from build123d import *

# Parameters (mm, degrees)
EXTRUDE_1_DEPTH          = 170
SKETCH_2_R               = 60
CUT_EXTRUDE_1_DEPTH      = 180
CUT_EXTRUDE_2_DEPTH      = 313.955268369
CUT_EXTRUDE_2_DEPTH_BACK = 313.955268369
SKETCH_3_R               = 30
FILLET_1_R               = 70
FILLET_2_R               = 20
FILLET_3_R               = 20


with BuildPart() as part:
    # 草图1 → 凸台-拉伸1 (new body)
    with BuildSketch(Plane.XY):
        Polygon((-180, 0), (0, 0), (0, -175), (8, -175), (8, 8), (-180, 8), (-188, 8), (-188, -175), (-180, -175), align=None)
    extrude(amount=EXTRUDE_1_DEPTH)

    # 草图2 → 切除-拉伸1 (cut)
    with BuildSketch(Plane(origin=(0, 8, 0), x_dir=(1, 0, 0), z_dir=(0, 1, 0))):
        with Locations(Location((-90, -85, 0), (0, 0, 180))):
            Circle(SKETCH_2_R)
    extrude(amount=-CUT_EXTRUDE_1_DEPTH, mode=Mode.SUBTRACT)

    # 草图3 → 切除-拉伸2 (cut, two sides: drawn at the far end of the back side and taken through both)
    with BuildSketch(Plane(origin=(8, 0, 0), x_dir=(0, 0, -1), z_dir=(1, 0, 0)).offset(-CUT_EXTRUDE_2_DEPTH_BACK)):
        with Locations(Location((-85, -95, 0), (0, 0, 90))):
            Circle(SKETCH_3_R)
    extrude(amount=CUT_EXTRUDE_2_DEPTH + CUT_EXTRUDE_2_DEPTH_BACK, mode=Mode.SUBTRACT)

    # 圆角1
    fillet_1_edges = [part.edges().sort_by_distance(p)[0] for p in [
        (4, -175, 0),
        (4, -175, 170),
        (-184, -175, 170),
        (-184, -175, 0),
    ]]
    fillet(fillet_1_edges, radius=FILLET_1_R)

    # 圆角2
    fillet_2_edges = [part.edges().sort_by_distance(p)[0] for p in [
        (0, 0, 85),
        (-180, 0, 85),
    ]]
    fillet(fillet_2_edges, radius=FILLET_2_R)

    # 圆角3
    fillet_3_edges = [part.edges().sort_by_distance(p)[0] for p in [
        (-188, 8, 85),
        (8, 8, 85),
    ]]
    fillet(fillet_3_edges, radius=FILLET_3_R)


solid = part.part
Build history of the part. All positions in model axes, mm. A direction names the side the tool comes from. Coordinates: 2 decimals unless noted, no trailing zeros. Order: outer loops, then holes, each group sorted by start corner. A loop starts at its lowest first (then second) coordinate and runs counter-clockwise, first axis right, second up. Notation, with made-up numbers: (61, -35) - (75, -35) arc R24 ccw to (75, -13) - close; hole circle Ø4 at (2, -3). An arc over 180 degrees is marked (long way). Write item = value, one per line. Start each with the question number.
1) Saw through at B-B on y = -95. Write the cut outline in (x, z), then the cut area to 3 significant figures.
2) Flat gauge pin, fed straight in: pin 1 Ø3 at (x, z) = (-150, 111.5) entering from -Y. Where does the tip first touch, or does it go through?
3) Saw through at C-C on y = -24. Write the cut outline in (x, z), then the cut area to 3 significant figures.
4) 3-axis set-ups, long thin cutter, end or side, ignore diameter. For faces 4 (the face through (-183.94, -153.95, 19.96)), 5 (the face through (-6.014, -5.703, 86.19)): which of +Z, -Z, +X, -X, +Y, -Y reach the whole face in a straight line?
5) Saw through at D-D on x = -90. Write the cut outline in (y, z), then the cut area to 3 significant figures.
6) Wall check: line 1 along Z through (x, y) = (-186, -95); line 2 along X through (y, z) = (-96, 120); line 3 along X through (y, z) = (-15.5, 33). Give the ranges that are in metal, low to high. Write a range as from..to.
7) Saw through at A-A on z = 85. Write the cut outline in (x, y).
8) Two-plate mould, pull along Y, no slides. Class faces 1 (the face through (-107, 0, 27)), 2 (the face through (-184.056, -117.111, 105.275)), 3 (the face through (0, -62, 84)): pulls with the +Y half, pulls with the -Y half, needs draft (parallel to the pull), parting line crosses it, or undercut.
From the geometry:
q1.outline = (-188, 0) - (-180, 0) - (-180, 55) - (-188, 55) - close; (-188, 115) - (-180, 115) - (-180, 170) - (-188, 170) - close; (0, 0) - (8, 0) - (8, 55) - (0, 55) - close; (0, 115) - (8, 115) - (8, 170) - (0, 170) - close
q1.area = 1,760 mm^2
q2.pin_1 = 0
q3.outline = (-188, 0) - (-180, 0) - (-180, 170) - (-188, 170) - close; (0, 0) - (8, 0) - (8, 170) - (0, 170) - close
q3.area = 2,720 mm^2
q4.face_4 = -Z, +X, -X, -Y
q4.face_5 = +Z, -Z, -Y
q5.outline = (0, 0) - (8, 0) - (8, 25) - (0, 25) - close; (0, 145) - (8, 145) - (8, 170) - (0, 170) - close
q5.area = 400 mm^2
q6.line_1 = 0..55, 115..170
q6.line_2 = -188..-180, 0..8
q6.line_3 = -188..-179.49, -0.51..8
q7.outline = (-188, -175) - (-180, -175) - (-180, -125) - (-188, -125) - close; (-188, -65) - (-180, -65) - (-180, -20) arc R20 cw to (-160, 0) - (-150, 0) - (-150, 8) - (-168, 8) arc R20 ccw to (-188, -12) - close; (-30, 0) - (-20, 0) arc R20 cw to (0, -20) - (0, -65) - (8, -65) - (8, -12) arc R20 ccw to (-12, 8) - (-30, 8) - close; (0, -175) - (8, -175) - (8, -125) - (0, -125) - close
q8.face_1 = pulls with the -Y half
q8.face_2 = undercut
q8.face_3 = needs draft
